Verification items for this drawing (mm, ordinates from the low corner). Round coordinates to 2 decimals unless told otherwise and drop trailing zeros. Write each loop counter-clockwise with the first axis right and the second up, starting at its lowest first coordinate (ties: lowest second). Pieces come first, ordered by that corner, then holes. Notation, with made-up numbers: (-7.75, 87) -> (11.25, 87) arc R26 cw to (11.25, 126) -> close; hole circle Ø2 at (24, -15). An arc over 180 degrees is marked (long way). Return JSON: item names as keys, results as strings. Group by question number.
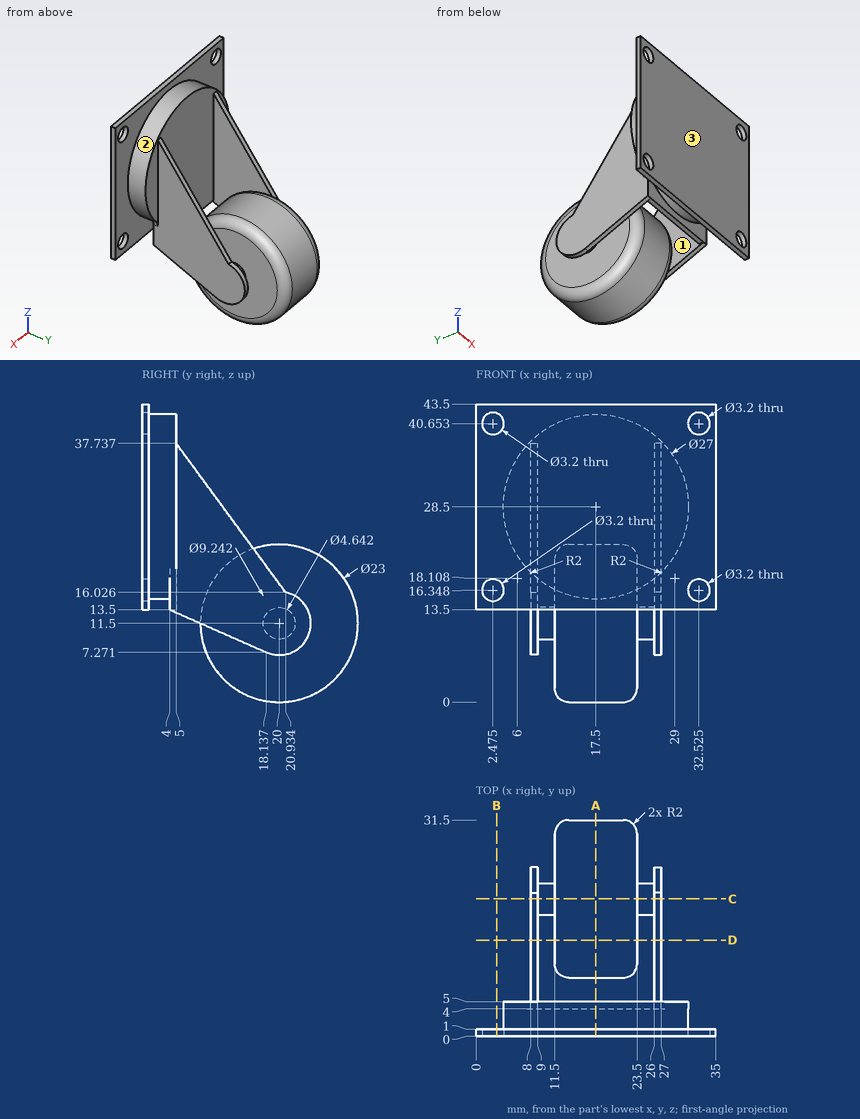
1) Go/stop test with flat-tipped pins: P1, Ø4, axis at y = 23.5, z = 25.5, coming from the -X side; P2, Ø3, axis at x = 12.5, z = 16.5, coming from the -Y side; P3, Ø10, axis at x = 17, y = 7.5, coming from the -Z side; P4, Ø10, axis at x = 5.5, z = 23, coming from the +Y side. Record where each tip stops, or that it passes through.
2) Sectioned sample at B-B on x = 3. Enter the section's corners in (y, z).
3) Sectioned sample at D-D on y = 14. State how many separate pieces and enclosed holes the cut face has, and give its area (3 significant figures).
4) Sectioned sample at A-A on x = 17.5. Enter the section's corners in (y, z).
5) Material ranges on probe 1 along X at (y, z) = (21, 9); probe 2 along X at (y, z) = (9, 21); probe 3 along Y at (x, z) = (5, 39.5), recorded low to high. Write a range as [from, to].
6) Mould release check, pull along X, two halves, no side actions. Record for the marked faces 1, 2 and 3: +X half, -X half, draft (parallel to the pull), parting line (faces both ways), or undercut.
7) Sectioned sample at C-C on y = 20. Enter the section's corners in (x, z), and give its area (3 significant figures).
Evaluation:
{
 "1": {"P1": "passes through", "P2": "stops at y = 0", "P3": "stops at z = 2.78", "P4": "stops at y = 18.99"},
 "2": {"outline": "(0, 13.5) -> (1, 13.5) -> (1, 14.84) -> (0, 14.84) -> close; (0, 17.86) -> (1, 17.86) -> (1, 39.14) -> (0, 39.14) -> close; (0, 42.16) -> (1, 42.16) -> (1, 43.5) -> (0, 43.5) -> close"},
 "3": {"separate pieces": "3", "enclosed holes": "0", "area": "264 mm2"},
 "4": {"outline": "(0, 13.5) -> (1, 13.5) -> (1, 15) -> (4, 15) -> (4, 13.5) -> (5, 13.5) -> (5, 42) -> (1, 42) -> (1, 43.5) -> (0, 43.5) -> close; circle Ø23 at (20, 11.5)"},
 "5": {"probe 1": "x = [8, 9], [11.5, 23.5], [26, 27]", "probe 2": "x = [8, 9], [26, 27]", "probe 3": "y = [0, 1]"},
 "6": {"face 1": "undercut", "face 2": "parting line", "face 3": "draft"},
 "7": {"outline": "(8, 6.88) -> (9, 6.88) -> (9, 9.18) -> (11.5, 9.18) -> (11.5, 2) arc R2 ccw to (13.5, 0) -> (21.5, 0) arc R2 ccw to (23.5, 2) -> (23.5, 9.18) -> (26, 9.18) -> (26, 6.88) -> (27, 6.88) -> (27, 17.3) -> (26, 17.3) -> (26, 13.82) -> (23.5, 13.82) -> (23.5, 21) arc R2 ccw to (21.5, 23) -> (13.5, 23) arc R2 ccw to (11.5, 21) -> (11.5, 13.82) -> (9, 13.82) -> (9, 17.3) -> (8, 17.3) -> close", "area": "317 mm2"}
}
